Geometry check sheet. Reference: the model listing, model coordinates, mm. Face numbers are marked on the shaded views. A direction names the side the tool comes from. Coordinates: 2 decimals unless noted, no trailing zeros. Write each loop counter-clockwise with the first axis right and the second up, starting at its lowest first coordinate (ties: lowest second). Pieces come first, ordered by that corner, then holes. Notation, with made-up numbers: (59.25, 6) -> (76.25, 6) arc R25 cw to (76.25, 36) -> close; hole circle Ø3 at (38.5, -20). An arc over 180 degrees is marked (long way). Answer in a Markdown table with one row per item. Add a question column.
1. Scan lines: L1, parallel to Z at x = 4.5, y = 0; L2, parallel to Y at x = 4.75, z = -0.5; L3, parallel to X at y = 0, z = 3. Record each from-to range of solid material in increasing order. Write a range as from..to.
2. Cross-section at A-A on x = 0.5. Record the cut outline in (y, z).
3. Mould release check, pull along Y, two halves, no side actions. Record for the marked faces 1, 2 and 3: pulls with the +Y half, pulls with the -Y half, needs draft (parallel to the pull), parting line crosses it, or undercut.
4. Depth check by flat-ended pin: P1, Ø4, axis at x = 4.5, z = 2, coming from the +Y side; P2, Ø3, axis at x = 2.5, y = -1, coming from the -Z side. Enter the tip coordinate at first touch or a pass-through.
5. Set-up check for the marked faces 4, 5 and 6: record each of +Z, -Z, +X, -X, +Y, -Y from which the full face is reachable in a straight line by a thin tool's end or side.
6. Cross-section at B-B on x = 7.75. Record the cut outline in (y, z).
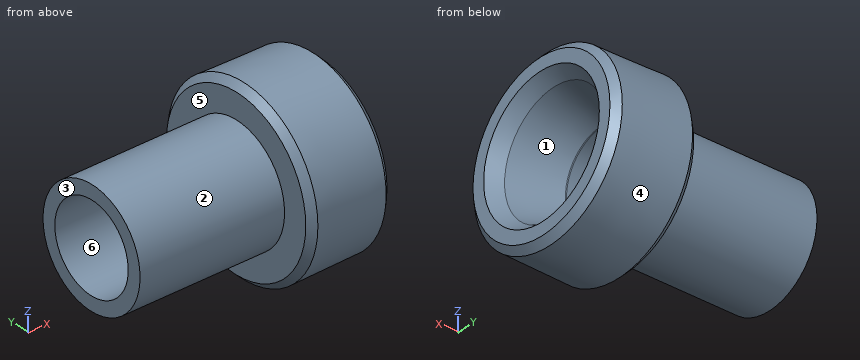
Autodesk Inventor part; units mm, degrees
ref_plane "YZ Plane" through (0, 0, 0) normal (1, 0, 0) x (0, 1, 0)
ref_plane "XZ Plane" through (0, 0, 0) normal (0, 1, 0) x (-1, 0, 0)
ref_plane "XY Plane" through (0, 0, 0) normal (0, 0, 1) x (1, 0, 0)
sketch "Sketch1" plane through (0, 0, 0) normal (0, 0, 1) x (1, 0, 0)
  line L0 (0, 1.651) -> (6.3575, 1.651)
  line L1 (6.3978, 1.6576) -> (8.2197, 2.2672)
  line L2 (8.2197, 2.2672) -> (8.7376, 2.6035)
  line L3 (8.7376, 2.6035) -> (8.7376, 3.0815)
  line L4 (8.4836, 3.3399) -> (5.8166, 3.3865)
  line L5 (5.5626, 3.1369) -> (5.5626, 2.1844)
  line L6 (5.5626, 2.1844) -> (0, 2.1844)
  line L7 (0, 2.1844) -> (0, 1.651)
  line L8 (5.8166, 3.3865) -> (5.5626, 3.1369)
  line L9 (8.4836, 3.3399) -> (8.7376, 3.0815)
  arc A0 (6.3575, 1.651) -> (6.3978, 1.6576) centre (6.3575, 1.778) ccw
  line L10 (-6.035, 0) -> (36.2102, 0)
  point P0 (0, 0)
  point P1 (8.7376, 3.3355)
  point P2 (5.5626, 3.3909)
  dimension "d0" = 18.5
  dimension "d1" = 33
  dimension "d2" = 89
  dimension "d3" = 3.3909
  dimension "d4" = 2.1844
  dimension "d5" = 1.651
  dimension "d6" = 8.7376
  dimension "d7" = 2.6035
  dimension "d8" = 2.2672
  dimension "d9" = 3.175
  dimension "d10" = 0.254
  dimension "d11" = 0.254
  dimension "d12" = 0.254
  dimension "d13" = 0.254
  dimension "d14" = 0.127
  dimension "d16" = 0.0066
revolve "Revolution1" add sketch "Sketch1" angle 360 about axis through (-10, 0, 0) along (1, 0, 0)
equation "\"d9\" = MS20819_J"
equation "\"d14\" = MS20819_R"
equation "\"MS20819_B\" = 3.302"
equation "\"MS20819_C\" = 4.3688"
equation "\"MS20819_F\" = 5.207"
equation "\"MS20819_G\" = 6.7818"
equation "\"MS20819_J\" = 3.175"
equation "\"MS20819_M\" = 8.7376"
equation "\"MS20819_N\" = 4.5212"
equation "\"MS20819_R\" = 0.127"
equation "\"Tube_OD\" = 3.175"
properties part number "MS20819-2D" material "Aluminum 2014-T6"
Results found:
| question | item | result |
|---|---|---|
| 1 | L1 | z = -2.18..-1.65, 1.65..2.18 |
| 1 | L2 | y = -2.13..-1.57, 1.57..2.13 |
| 1 | L3 | x = 5.56..8.74 |
| 2 | outline | circle Ø4.37 at (0, 0); hole circle Ø3.3 at (0, 0) |
| 3 | face 1 | undercut |
| 3 | face 2 | parting line crosses it |
| 3 | face 3 | needs draft |
| 4 | P1 | stops at y = 3.35 |
| 4 | P2 | stops at z = -2.18 |
| 5 | face 4 | +X |
| 5 | face 5 | -X |
| 5 | face 6 | +X, -X |
| 6 | outline | circle Ø6.71 at (0, 0); hole circle Ø4.22 at (0, 0) |
